The listing builds one solid part. Answer for the finished solid, in the listing's coordinates (mm). Face numbers are marked on the shaded views. A direction names the side the tool comes from. Give positions to 0.01 mm unless a question says otherwise; leave off trailing zeros. Order: outer loops, then holes, each group sorted by start corner. A loop starts at its lowest first (then second) coordinate and runs counter-clockwise, first axis right, second up.
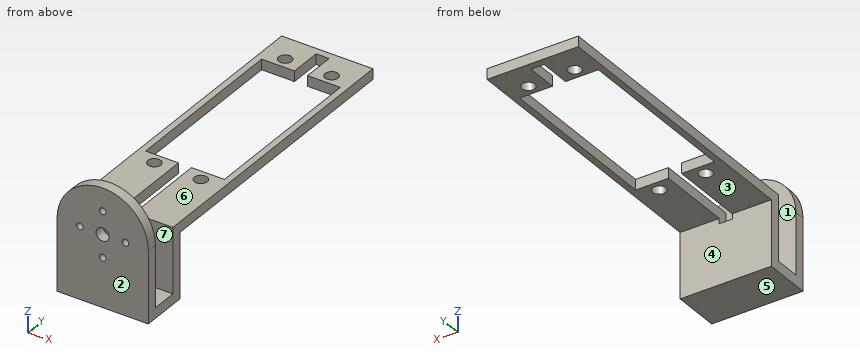
```python
from build123d import *

# Parameters (mm, degrees)
BOSS_EXTRUDE2_DEPTH = 4
SKETCH4_W           = 35
SKETCH4_H           = 4
BOSS_EXTRUDE3_DEPTH = 10
BOSS_EXTRUDE4_DEPTH = 35
SKETCH9_R           = 2.5
CUT_EXTRUDE1_DEPTH  = 6
SKETCH10_R          = 1.25
CUT_EXTRUDE2_DEPTH  = 6
SKETCH11_R          = 2.5
CUT_EXTRUDE3_DEPTH  = 4


with BuildPart() as part:
    # Sketch3 → Boss-Extrude2 (new body)
    with BuildSketch(Plane(origin=(0, 0, 0), x_dir=(1, 0, 0), z_dir=(0, 1, 0))):
        with BuildLine():
            Line((-17.5, 0), (-17.5, 27.5))
            Line((-17.5, 27.5), (17.5, 27.5))
            Line((17.5, 27.5), (17.5, 0))
            ThreePointArc((17.5, 0), (0, -17.5), (-17.5, 0))
        make_face()
    extrude(amount=BOSS_EXTRUDE2_DEPTH)

    # Sketch4 → Boss-Extrude3 (add)
    with BuildSketch(Plane(origin=(0, 4, 0), x_dir=(1, 0, 0), z_dir=(0, 1, 0))):
        with Locations((0, 25.5)):
            Rectangle(SKETCH4_W, SKETCH4_H)
    extrude(amount=BOSS_EXTRUDE3_DEPTH)

    # Sketch6 → Boss-Extrude4 (add)
    with BuildSketch(Plane.ZY.offset(17.5)):
        Polygon((-27.5, 14), (-27.5, 18), (-2.5, 18), (-2.5, 128), (1.5, 128), (1.5, 14), align=None)
    extrude(amount=-BOSS_EXTRUDE4_DEPTH)

    # Sketch9 → Cut-Extrude1 (cut)
    with BuildSketch(Plane.XY.offset(1.5)):
        with Locations((-8.9, 117.2)):
            Circle(SKETCH9_R)
        with Locations((8.9, 117.2)):
            Circle(SKETCH9_R)
        with Locations((-8.9, 42.7)):
            Circle(SKETCH9_R)
        with Locations((8.9, 42.7)):
            Circle(SKETCH9_R)
        Polygon((-15.1, 113), (-2.5, 113), (-2.5, 125.287895972), (0, 125.287895972), (2.5, 125.287895972), (2.5, 113), (15.1, 113), (15.1, 46.9), (2.5, 46.9), (2.5, 10), (-2.5, 10), (-2.5, 46.9), (-15.1, 46.9), align=None)
    extrude(amount=-CUT_EXTRUDE1_DEPTH, mode=Mode.SUBTRACT)

    # Sketch10 → Cut-Extrude2 (cut)
    with BuildSketch(Plane.XZ):
        with Locations((-8.75, 0)):
            Circle(SKETCH10_R)
        with Locations((8.75, 0)):
            Circle(SKETCH10_R)
        with Locations((0, 8.75)):
            Circle(SKETCH10_R)
        with Locations((0, -8.75)):
            Circle(SKETCH10_R)
    extrude(amount=-CUT_EXTRUDE2_DEPTH, mode=Mode.SUBTRACT)

    # Sketch11 → Cut-Extrude3 (cut)
    with BuildSketch(Plane.XZ):
        Circle(SKETCH11_R)
    extrude(amount=-CUT_EXTRUDE3_DEPTH, mode=Mode.SUBTRACT)


solid = part.part
```
1) A tool of negligible diameter and unlimited length cuts with its end or side. For the marked faces 5, 6 and 7, from which of +Z, -Z, +X, -X, +Y, -Y can it reach the whole face along a straight path? Write none if from no direction.
Geometry says:
face 5: -Z, +X, -X, +Y, -Y
face 6: +Z, +X, -X, +Y
face 7: +Z, +X, -X
2) Find section C-C (x = 0). Write down the section's boundary in (y, z), then the cut area to 3 significant figures.
Geometry says:
outline: (0, -27.5) - (18, -27.5) - (18, -4.5) - (14, -4.5) - (14, -23.5) - (4, -23.5) - (4, -10) - (0, -10) - close; (0, -7.5) - (4, -7.5) - (4, -2.5) - (0, -2.5) - close; (0, 2.5) - (4, 2.5) - (4, 7.5) - (0, 7.5) - close; (0, 10) - (4, 10) - (4, 17.5) - (0, 17.5) - close; (125.29, -2.5) - (128, -2.5) - (128, 1.5) - (125.29, 1.5) - close
area: 283 mm2
3) For a pull along Y with two mould halves and no side action, classify the marked faces 1, 2, 3 and 4 as +Y half, -Y half, draft (parallel to the pull), parting line (faces both ways), or undercut.
Geometry says:
face 1: undercut
face 2: -Y half
face 3: draft
face 4: +Y half
4) Given P1, Ø12, axis at x = 12.5, y = 32, coming from the -Z side; P2, Ø4, axis at x = 8.9, y = 42.7, coming from the +Z side; P3, Ø2, axis at x = 0, z = -8.75, coming from the +Y side; P4, Ø17.5, axis at x = -8, y = 75, coming from the +Z side, each flat-ended and moving along its own axis, determine where each tip first touches the part or whether it passes through.
Geometry says:
P1: stops at z = -2.5
P2: passes through
P3: stops at y = 18
P4: stops at z = 1.5
5) Find section B-B (y = 23). Write down the section's boundary in (x, z), then the cut area to 3 significant figures.
Geometry says:
outline: (-17.5, -2.5) - (-2.5, -2.5) - (-2.5, 1.5) - (-17.5, 1.5) - close; (2.5, -2.5) - (17.5, -2.5) - (17.5, 1.5) - (2.5, 1.5) - close
area: 120 mm2
6) Find section D-D (z = -8.75). Write down the section's boundary in (x, y), then the cut area to 3 significant figures.
Geometry says:
outline: (-17.5, 0) - (-1.25, 0) - (-1.25, 4) - (-17.5, 4) - close; (-17.5, 14) - (17.5, 14) - (17.5, 18) - (-17.5, 18) - close; (1.25, 0) - (17.5, 0) - (17.5, 4) - (1.25, 4) - close
area: 270 mm2
7) Find section A-A (y = 42.7). Write down the section's boundary in (x, z).
Geometry says:
outline: (-17.5, -2.5) - (-11.4, -2.5) - (-11.4, 1.5) - (-17.5, 1.5) - close; (-6.4, -2.5) - (-2.5, -2.5) - (-2.5, 1.5) - (-6.4, 1.5) - close; (2.5, -2.5) - (6.4, -2.5) - (6.4, 1.5) - (2.5, 1.5) - close; (11.4, -2.5) - (17.5, -2.5) - (17.5, 1.5) - (11.4, 1.5) - close
8) Straight lines are drawn through the part: probe 1 along Y at (x, z) = (-8.9, -0.95); probe 2 along Z at (x, y) = (0, 2.55); probe 3 along X at (y, z) = (42, 0). For each, find the intervals that lie inside material, in ascending order.
Geometry says:
probe 1: y = 14 to 40.2, 45.2 to 46.9, 113 to 114.7, 119.7 to 128
probe 2: z = -27.5 to -10, -7.5 to -2.5, 2.5 to 7.5, 10 to 17.5
probe 3: x = -17.5 to -11.3, -6.5 to -2.5, 2.5 to 6.5, 11.3 to 17.5
